CAD build for the part. Positions are in the model's coordinates, mm. Face numbers are marked on the shaded views. A direction names the side the tool comes from. Give positions to 0.01 mm unless a question says otherwise; leave off trailing zeros. Loops run counter-clockwise (first coordinate to the right, second up) from the corner with the lowest first, then second, coordinate; pieces in that order, holes last.
Item 1: Probe probe 1 along Y at (x, z) = (18, 23); probe 2 along Y at (x, z) = (18, 19.75); probe 3 along Z at (x, y) = (11, 42). List the from-to ranges inside material, lowest first.
Item 2: Saw through at B-B on x = 18. Give the cut face in (y, z).
Item 3: Saw through at A-A on y = -50.2. Give the cut face in (x, z).
Item 4: Saw through at C-C on z = -1.5. Give the cut face in (x, y), plus the area to 3 significant figures.
Item 5: Which spindle directions (+Z, -Z, +X, -X, +Y, -Y) get a long thin tool onto all of the face, cutting with end or side? Do the marked faces 1, 2 and 3. Say none if no direction does.
Item 6: Saw through at D-D on x = 33.5. Give the cut face in (y, z), plus the area to 3 significant figures.
Item 7: Drop flat-ended pins along their axis: P1, Ø5.5, axis at x = 12.5, y = 47, coming from the -Z side; P2, Ø2, axis at x = 8, z = -17, coming from the +Y side; P3, Ø2, axis at x = 27.5, z = 16.5, coming from the -Y side. Give the stop position or say it passes through.
from build123d import *

# Parameters (mm, degrees)
F1_DEPTH = 36
F2_R     = 3.1
F3_DEPTH = 8.001
F4_SIZE  = 7
F5_R     = 3


with BuildPart() as f1:
    # F0 (on Right) → F1 (new body)
    with BuildSketch(Plane.YZ):
        with BuildLine():
            Line((-16, 26), (-26, 26))
            Line((-26, 26), (-59.2, 26))
            Line((-59.2, 26), (-59.2, 18))
            Line((-59.2, 18), (-34.2, 18))
            Line((-34.2, 18), (-34.2, 0))
            ThreePointArc((-34.2, 0), (0, -34.2), (34.2, 0))
            Line((34.2, 0), (34.2, 18))
            Line((34.2, 18), (59.2, 18))
            Line((59.2, 18), (59.2, 26))
            Line((59.2, 26), (26, 26))
            Line((26, 26), (16, 26))
            Line((16, 26), (16, 20.493902))
            ThreePointArc((16, 20.493902), (23.366643, 11.401754), (26, 0))
            ThreePointArc((26, 0), (0, -26), (-26, 0))
            ThreePointArc((-26, 0), (-23.366643, 11.401754), (-16, 20.493902))
            Line((-16, 20.493902), (-16, 26))
        make_face()
    extrude(amount=F1_DEPTH)

    # F2 (on face) → F3 (cut, through all)
    with BuildSketch(Plane(origin=(0, 0, 18), x_dir=(1, 0, 0), z_dir=(0, 0, -1))):
        with Locations((18, 50.2)):
            Circle(F2_R)
        with Locations((18, -50.2)):
            Circle(F2_R)
    extrude(amount=-F3_DEPTH, mode=Mode.SUBTRACT)

    # F4
    f4_edges = [f1.edges().sort_by_distance(p)[0] for p in [
        (18, -34.2, 18),
        (18, 34.2, 18),
    ]]
    chamfer(f4_edges, length=F4_SIZE)

    # F5
    f5_edges = [f1.edges().sort_by_distance(p)[0] for p in [
        (18, 16, 20.493902),
        (18, -16, 20.493902),
    ]]
    fillet(f5_edges, radius=F5_R)


solid = f1.part
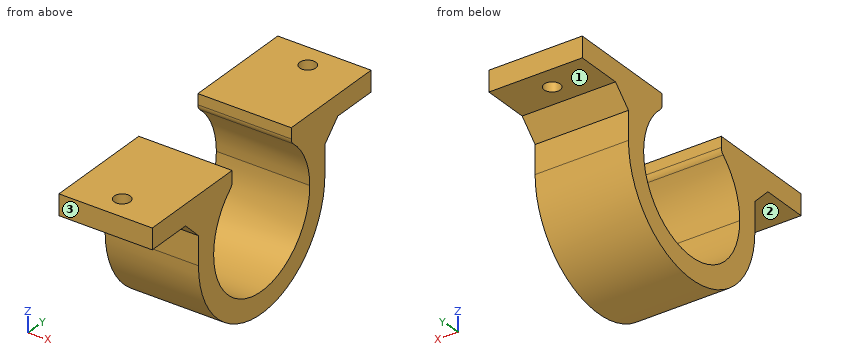
Results below:
1. probe 1: y = -59.2 to -53.3, -47.1 to -16, 16 to 47.1, 53.3 to 59.2
1. probe 2: y = -59.2 to -53.3, -47.1 to -16.92, 16.92 to 47.1, 53.3 to 59.2
1. probe 3: z = 18 to 26
2. outline: (-59.2, 18) - (-53.3, 18) - (-53.3, 26) - (-59.2, 26) - close; (-47.1, 18) - (-41.2, 18) - (-34.2, 11) - (-34.2, 0) arc R34.2 ccw to (34.2, 0) - (34.2, 11) - (41.2, 18) - (47.1, 18) - (47.1, 26) - (16, 26) - (16, 21.91) arc R3 ccw to (17.03, 19.64) arc R26 cw to (26, 0) arc R26 cw to (-26, 0) arc R26 cw to (-17.03, 19.64) arc R3 ccw to (-16, 21.91) - (-16, 26) - (-47.1, 26) - close; (53.3, 18) - (59.2, 18) - (59.2, 26) - (53.3, 26) - close
3. outline: (0, 18) - (14.9, 18) - (14.9, 26) - (0, 26) - close; (21.1, 18) - (36, 18) - (36, 26) - (21.1, 26) - close
4. outline: (0, -34.17) - (36, -34.17) - (36, -25.96) - (0, -25.96) - close; (0, 25.96) - (36, 25.96) - (36, 34.17) - (0, 34.17) - close
4. area: 591 mm2
5. face 1: -Z, +X, -X, +Y
5. face 2: -Z, +X, -X, -Y
5. face 3: +Z, -Z, +X, -X, -Y
6. outline: (-59.2, 18) - (-41.2, 18) - (-34.2, 11) - (-34.2, 0) arc R34.2 ccw to (34.2, 0) - (34.2, 11) - (41.2, 18) - (59.2, 18) - (59.2, 26) - (16, 26) - (16, 21.91) arc R3 ccw to (17.03, 19.64) arc R26 cw to (26, 0) arc R26 cw to (-26, 0) arc R26 cw to (-17.03, 19.64) arc R3 ccw to (-16, 21.91) - (-16, 26) - (-59.2, 26) - close
6. area: 1,880 mm2
7. P1: stops at z = 18
7. P2: stops at y = 30.23
7. P3: stops at y = -40.7
